from build123d import *

# Parameters (mm, degrees)
SKETCH1_W           = 18
SKETCH1_H           = 4.7
BOSS_EXTRUDE1_DEPTH = 1.5
SKETCH2_W           = 5
SKETCH2_H           = 0.9
SKETCH2_W_2         = 18
SKETCH2_H_2         = 2.5
BOSS_EXTRUDE2_DEPTH = 4.5
SKETCH3_W           = 18
SKETCH3_H           = 2.5
BOSS_EXTRUDE3_DEPTH = 4
SKETCH4_W           = 4.7
SKETCH4_H           = 10
BOSS_EXTRUDE4_DEPTH = 1.5
SKETCH5_W           = 4.7
SKETCH5_H           = 10
BOSS_EXTRUDE5_DEPTH = 1.5
SKETCH6_W           = 21
SKETCH6_H           = 1.5
BOSS_EXTRUDE6_DEPTH = 8


with BuildPart() as part:
    # Sketch1 → Boss-Extrude1 (new body)
    with BuildSketch(Plane(origin=(0, 0, 0), x_dir=(1, 0, 0), z_dir=(0, 1, 0))):
        with Locations((5.918454936, -0.847854077)):
            Rectangle(SKETCH1_W, SKETCH1_H)
    extrude(amount=BOSS_EXTRUDE1_DEPTH)

    # Sketch2 → Boss-Extrude2 (add)
    with BuildSketch(Plane(origin=(0, 1.5, 0), x_dir=(1, 0, 0), z_dir=(0, 1, 0))):
        with Locations((-0.581545064, 1.052145923)):
            Rectangle(SKETCH2_W, SKETCH2_H)
        with Locations((12.418454936, 1.052145923)):
            Rectangle(SKETCH2_W, SKETCH2_H)
        with Locations((5.918454936, -1.947854077)):
            Rectangle(SKETCH2_W_2, SKETCH2_H_2)
    extrude(amount=BOSS_EXTRUDE2_DEPTH)

    # Sketch3 → Boss-Extrude3 (add)
    with BuildSketch(Plane(origin=(0, 6, 0), x_dir=(1, 0, 0), z_dir=(0, 1, 0))):
        with Locations((5.918454936, -1.947854077)):
            Rectangle(SKETCH3_W, SKETCH3_H)
    extrude(amount=BOSS_EXTRUDE3_DEPTH)

    # Sketch4 → Boss-Extrude4 (add)
    with BuildSketch(Plane(origin=(14.918454936, 0, 0), x_dir=(0, 0, -1), z_dir=(1, 0, 0))):
        with Locations((-0.847854077, 5)):
            Rectangle(SKETCH4_W, SKETCH4_H)
    extrude(amount=BOSS_EXTRUDE4_DEPTH)

    # Sketch5 → Boss-Extrude5 (add)
    with BuildSketch(Plane.ZY.offset(3.081545064)):
        with Locations((0.847854077, 5)):
            Rectangle(SKETCH5_W, SKETCH5_H)
    extrude(amount=BOSS_EXTRUDE5_DEPTH)

    # Sketch6 → Boss-Extrude6 (add)
    with BuildSketch(Plane.XY.offset(3.197854077)):
        with Locations((5.918454936, 0.75)):
            Rectangle(SKETCH6_W, SKETCH6_H)
    extrude(amount=BOSS_EXTRUDE6_DEPTH)


solid = part.part
Here's how the part is built. I have some questions about the finished solid (model axes, mm). A direction names the side the tool comes from. Give positions to 0.01 mm unless a question says otherwise; leave off trailing zeros. Order: outer loops, then holes, each group sorted by start corner. A loop starts at its lowest first (then second) coordinate and runs counter-clockwise, first axis right, second up. Notation, with made-up numbers: (19.5, 67) -> (56.5, 67) arc R6 cw to (56.5, 72) -> close; hole circle Ø11 at (-26.75, 42). An arc over 180 degrees is marked (long way). One line per item, written item: value. Start each with the question number.
1. We'd pull the mould along Z, two halves only. Please class faces 6 (the face through (6, 0, 5)), 7 (the face through (14.918, 7, 0)), 8 (the face through (6, 6, 3.198)): released by +Z, released by -Z, zero draft, split by the parting line, or undercut.
2. Imagine slicing it at D-D, the plane y = 6.5. List the corners of the cut face in (x, z) for me.
3. For faces 1 (the face through (6, 1.5, 7)), 2 (the face through (9.918, 4, -1)), 3 (the face through (6, 1, 11.198)), 4 (the face through (6, 6, 0.698)), 5 (the face through (-4.582, 4, 2)), which set-ups out of +Z, -Z, +X, -X, +Y, -Y let a thin tool reach every point of the face, with its end or its side?
4. Imagine slicing it at B-B, the plane x = 3.25. List the corners of the cut face in (y, z) for me.
5. Will these pins go through, and if not, where does the flat tip stop? pin 1 Ø1.1 at (x, z) = (2, -1) entering from +Y; pin 2 Ø1.5 at (x, y) = (9, 2.5) entering from -Z; pin 3 Ø4 at (x, y) = (6, 4.5) entering from +Z.
6. Imagine slicing it at C-C, the plane z = 5. List the corners of the cut face in (x, y) for me.
7. Imagine slicing it at A-A, the plane y = 3.5. List the corners of the cut face in (x, z) for me, plus the area to 3 significant figures.
8. I need wall thicknesses on probe 1 along Z at (x, y) = (11.5, 3); probe 2 along X at (y, z) = (9.75, 0); probe 3 along Y at (x, z) = (2.25, -1). Which ranges of each line are inside material? Lowest first, please. Write a range as from..to.
Values follow:
1. face 6: zero draft
1. face 7: undercut
1. face 8: released by +Z
2. outline: (-4.58, -1.5) -> (-3.08, -1.5) -> (-3.08, 0.7) -> (14.92, 0.7) -> (14.92, -1.5) -> (16.42, -1.5) -> (16.42, 3.2) -> (-4.58, 3.2) -> close
3. face 1: +Z, +X, -X, +Y
3. face 2: -Z, +Y
3. face 3: +Z, +X, -X, +Y, -Y
3. face 4: +Y
3. face 5: +Z, -Z, -X, +Y, -Y
4. outline: (0, -1.5) -> (1.5, -1.5) -> (1.5, 0.7) -> (10, 0.7) -> (10, 3.2) -> (1.5, 3.2) -> (1.5, 11.2) -> (0, 11.2) -> close
5. pin 1: stops at y = 6
5. pin 2: stops at z = 0.7
5. pin 3: stops at z = 3.2
6. outline: (-4.58, 0) -> (16.42, 0) -> (16.42, 1.5) -> (-4.58, 1.5) -> close
7. outline: (-4.58, -1.5) -> (1.92, -1.5) -> (1.92, -0.6) -> (-3.08, -0.6) -> (-3.08, 0.7) -> (14.92, 0.7) -> (14.92, -0.6) -> (9.92, -0.6) -> (9.92, -1.5) -> (16.42, -1.5) -> (16.42, 3.2) -> (-4.58, 3.2) -> close
7. area: 68.1 mm2
8. probe 1: z = -1.5..-0.6, 0.7..3.2
8. probe 2: x = -4.58..-3.08, 14.92..16.42
8. probe 3: y = 0..1.5
